Drawing for the job (mm, zero at the part's lowest x, y, z). A direction names the side the tool comes from. Round coordinates to 2 decimals unless told otherwise and drop trailing zeros. Order: outer loops, then holes, each group sorted by start corner. A loop starts at its lowest first (then second) coordinate and runs counter-clockwise, first axis right, second up. Notation, with made-up numbers: (82, 50) - (132, 50) arc R27 cw to (132, 69) - close; hole circle Ø5 at (24, -22). An arc over 180 degrees is marked (long way). Put each result on its own line as item: value. Start each with the question number.
Item 1: Probe probe 1 along Y at (x, z) = (66, 6); probe 2 along X at (y, z) = (72, 3); probe 3 along Y at (x, z) = (4, 16.5). List the from-to ranges inside material, lowest first.
Item 2: Mould opens along Y. For the marked faces 6, 7 and 8 say: pulls with the +Y half, pulls with the -Y half, needs draft (parallel to the pull), parting line crosses it, or undercut.
Item 3: Saw through at C-C on z = 4. List the corners of the cut face in (x, y), plus the area to 3 significant figures.
Item 4: Pin check, flat tips, straight feed: pin 1 Ø7 at (x, y) = (66, 72) entering from +Z; pin 2 Ø24 at (x, y) = (68, 36) entering from +Z; pin 3 Ø5 at (x, z) = (18, 24.5) entering from -Y; pin 4 Ø5 at (y, z) = (65.5, 5) entering from -X. Stop position of each tip, or through.
Item 5: Which spindle directions (+Z, -Z, +X, -X, +Y, -Y) get a long thin tool onto all of the face, cutting with end or side? Do the marked faces 1, 2, 3, 4 and 5. Say none if no direction does.
Item 6: Saw through at B-B on z = 32. List the corners of the cut face in (x, y), plus the area to 3 significant figures.
Item 7: Saw through at D-D on z = 11. List the corners of the cut face in (x, y).
Item 8: Saw through at A-A on x = 66. List the corners of the cut face in (y, z), plus the area to 3 significant figures.
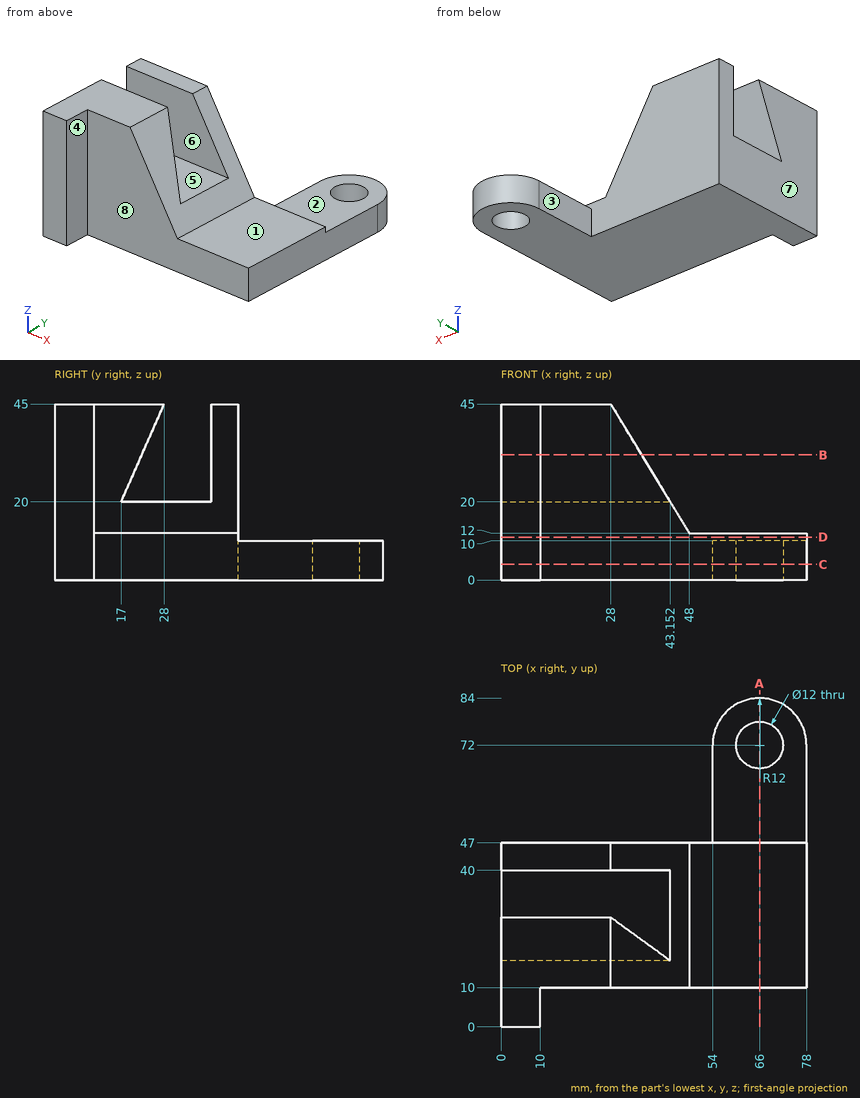
Results found:
1. probe 1: y = 10 to 66, 78 to 84
1. probe 2: x = 54 to 60, 72 to 78
1. probe 3: y = 0 to 47
2. face 6: undercut
2. face 7: needs draft
2. face 8: pulls with the -Y half
3. outline: (0, 0) - (10, 0) - (10, 10) - (78, 10) - (78, 72) arc R12 ccw to (54, 72) - (54, 47) - (0, 47) - close; hole circle Ø12 at (66, 72)
3. area: 3,700 mm²
4. pin 1: passes through
4. pin 2: stops at z = 12
4. pin 3: stops at y = 10
4. pin 4: stops at x = 54
5. face 1: +Z, +X, +Y, -Y
5. face 2: +Z, +X, -X, +Y
5. face 3: +Z, -Z, -X, +Y
5. face 4: +Z, -Z, +X, -Y
5. face 5: +X, -X
6. outline: (0, 0) - (10, 0) - (10, 10) - (35.88, 10) - (35.88, 22.28) - (0, 22.28) - close; (0, 40) - (35.88, 40) - (35.88, 47) - (0, 47) - close
6. area: 792 mm²
7. outline: (0, 0) - (10, 0) - (10, 10) - (78, 10) - (78, 47) - (0, 47) - close
8. outline: (10, 0) - (66, 0) - (66, 10) - (47, 10) - (47, 12) - (10, 12) - close; (78, 0) - (84, 0) - (84, 10) - (78, 10) - close
8. area: 694 mm²
